from build123d import *

# Parameters (mm, degrees)
SKETCH1_R           = 12.7
SKETCH1_R_2         = 3.175
SKETCH1_R_3         = 2.07
BOSS_EXTRUDE1_DEPTH = 1.5
FILLET1_R           = 3.000000096
CUT_EXTRUDE1_START  = -3
CUT_EXTRUDE1_DEPTH  = 3


with BuildPart() as part:
    # Sketch1 → Boss-Extrude1 (new, symmetric)
    with BuildSketch(Plane.XY):
        Polygon((-19.05, 82.55), (19.05, 82.55), (25.4, 57.15), (25.4, -19.05), (-25.4, -19.05), (-25.4, 57.15), align=None)
        Circle(SKETCH1_R, mode=Mode.SUBTRACT)
        with Locations((-19.05, -12.7)):
            Circle(SKETCH1_R_2, mode=Mode.SUBTRACT)
        with Locations((19.05, 12.7)):
            Circle(SKETCH1_R_2, mode=Mode.SUBTRACT)
        with Locations((-19.05, 12.7)):
            Circle(SKETCH1_R_3, mode=Mode.SUBTRACT)
        with Locations((19.05, -12.7)):
            Circle(SKETCH1_R_3, mode=Mode.SUBTRACT)
        with Locations((0, 57.15)):
            Circle(SKETCH1_R_2, mode=Mode.SUBTRACT)
        with Locations((12.7, 25.4)):
            Circle(SKETCH1_R_3, mode=Mode.SUBTRACT)
        with Locations((12.7, 38.1)):
            Circle(SKETCH1_R_3, mode=Mode.SUBTRACT)
        with Locations((12.7, 50.8)):
            Circle(SKETCH1_R_3, mode=Mode.SUBTRACT)
        with Locations((12.7, 63.5)):
            Circle(SKETCH1_R_3, mode=Mode.SUBTRACT)
        with Locations((12.7, 76.2)):
            Circle(SKETCH1_R_3, mode=Mode.SUBTRACT)
        with Locations(Location((-12.7, 25.4, 0), (0, 0, 180))):
            Circle(SKETCH1_R_3, mode=Mode.SUBTRACT)
        with Locations(Location((-12.7, 38.1, 0), (0, 0, 180))):
            Circle(SKETCH1_R_3, mode=Mode.SUBTRACT)
        with Locations(Location((-12.7, 50.8, 0), (0, 0, 180))):
            Circle(SKETCH1_R_3, mode=Mode.SUBTRACT)
        with Locations(Location((-12.7, 63.5, 0), (0, 0, 180))):
            Circle(SKETCH1_R_3, mode=Mode.SUBTRACT)
        with Locations(Location((-12.7, 76.2, 0), (0, 0, 180))):
            Circle(SKETCH1_R_3, mode=Mode.SUBTRACT)
    extrude(amount=BOSS_EXTRUDE1_DEPTH, both=True)

    # Fillet1
    fillet1_edges = [part.edges().sort_by_distance(p)[0] for p in [
        (-19.05, 82.55, 0),
        (19.05, 82.55, 0),
        (25.4, 57.15, 0),
        (25.4, -19.05, 0),
        (-25.4, -19.05, 0),
        (-25.4, 57.15, 0),
    ]]
    fillet(fillet1_edges, radius=FILLET1_R)

    # Sketch2 → Cut-Extrude1 (cut)
    with BuildSketch(Plane.XY.offset(1.5).offset(CUT_EXTRUDE1_START)):
        with BuildLine():
            Line((5.08, 17.78), (-5.08, 17.78))
            Line((-5.08, 17.78), (-5.08, 11.639742265))
            ThreePointArc((-5.08, 11.639742265), (0, 12.7), (5.08, 11.639742265))
            Line((5.08, 11.639742265), (5.08, 17.78))
        make_face()
        Polygon((0, -17.05), (-1, -19.05), (1, -19.05), align=None)
        Polygon((1, 82.55), (-1, 82.55), (0, 80.55), align=None)
    extrude(amount=CUT_EXTRUDE1_DEPTH, mode=Mode.SUBTRACT)


solid = part.part
Verification items for the finished model (mm, model axes). A direction names the side the tool comes from. Coordinates: 2 decimals unless noted, no trailing zeros. Write each loop counter-clockwise with the first axis right and the second up, starting at its lowest first coordinate (ties: lowest second). Pieces come first, ordered by that corner, then holes. Notation, with made-up numbers: (-32.5, 18) -> (-7.5, 18) arc R32 ccw to (-7.5, 48) -> close; hole circle Ø5 at (-33, -29). An arc over 180 degrees is marked (long way). One line per item, written item: value. Start each with the question number.
Q1. Cross-section at A-A on y = 0. Enter the section's corners in (x, z).
Q2. Thickness scan on L1, parallel to X at y = 57, z = 0.55; L2, parallel to Y at x = -13, z = 0.75; L3, parallel to X at y = 0, z = 0.55. Record the ranges inside material, lowest first. Write a range as from..to.
Q3. Cross-section at B-B on y = 50.8. Enter the section's corners in (x, z).
Q4. Cross-section at D-D on x = 18. Enter the section's corners in (y, z), and give its area (3 significant figures).
Q5. Go/stop test with flat-tipped pins: P1, Ø5, axis at x = 12.7, y = 38.1, coming from the -Z side; P2, Ø4, axis at x = -19.05, y = -12.7, coming from the -Z side. Record where each tip stops, or that it passes through.
Q6. Access from +Z, -Z, +X, -X, +Y, -Y to the whole of each face (thin tool, end or side, straight path). Record for faces 1 (the flat face through (-25.4, 20, 0)), 2 (the flat face through (-5.08, 15, 0)).
Q7. Cross-section at C-C on x = 9.5. Enter the section's corners in (y, z).
Q8. Mould release check, pull along Y, two halves, no side actions. Record for faces 3 (the cylindrical face through (-13.813, 49.055, -0.021)), 4 (the flat face through (25.4, 21, 0)), 5 (the cylindrical face through (-24.5, -18.19, 0.02)): pulls with the +Y half, pulls with the -Y half, needs draft (parallel to the pull), parting line crosses it, or undercut.
Checked values:
1. outline: (-25.4, -1.5) -> (-12.7, -1.5) -> (-12.7, 1.5) -> (-25.4, 1.5) -> close; (12.7, -1.5) -> (25.4, -1.5) -> (25.4, 1.5) -> (12.7, 1.5) -> close
2. L1: x = -25.39..-3.17, 3.17..25.39
2. L2: y = -19.05..23.35, 27.45..36.05, 40.15..48.75, 52.85..61.45, 65.55..74.15, 78.25..82.55
2. L3: x = -25.4..-12.7, 12.7..25.4
3. outline: (-25.4, -1.5) -> (-14.77, -1.5) -> (-14.77, 1.5) -> (-25.4, 1.5) -> close; (-10.63, -1.5) -> (10.63, -1.5) -> (10.63, 1.5) -> (-10.63, 1.5) -> close; (14.77, -1.5) -> (25.4, -1.5) -> (25.4, 1.5) -> (14.77, 1.5) -> close
4. outline: (-19.05, -1.5) -> (-14.48, -1.5) -> (-14.48, 1.5) -> (-19.05, 1.5) -> close; (-10.92, -1.5) -> (9.7, -1.5) -> (9.7, 1.5) -> (-10.92, 1.5) -> close; (15.7, -1.5) -> (82.26, -1.5) -> (82.26, 1.5) -> (15.7, 1.5) -> close
4. area: 275 mm²
5. P1: stops at z = -1.5
5. P2: passes through
6. face 1: +Z, -Z, -X, +Y, -Y
6. face 2: +Z, -Z
7. outline: (-19.05, -1.5) -> (-8.43, -1.5) -> (-8.43, 1.5) -> (-19.05, 1.5) -> close; (8.43, -1.5) -> (82.55, -1.5) -> (82.55, 1.5) -> (8.43, 1.5) -> close
8. face 3: undercut
8. face 4: needs draft
8. face 5: pulls with the -Y half
